Input: part model. Units: mm. Frame: model coordinates. Face numbers are marked on the shaded views. A direction names the side the tool comes from. Round coordinates to 2 decimals unless told otherwise and drop trailing zeros. Order: outer loops, then holes, each group sorted by start corner. A loop starts at its lowest first (then second) coordinate and runs counter-clockwise, first axis right, second up. Notation, with made-up numbers: (-22.5, -22) -> (-0.5, -22) arc R23 ccw to (-0.5, 13) -> close; hole circle Ø5 at (89.5, 81.5). An arc over 180 degrees is marked (long way). Use a Markdown table: item, result.
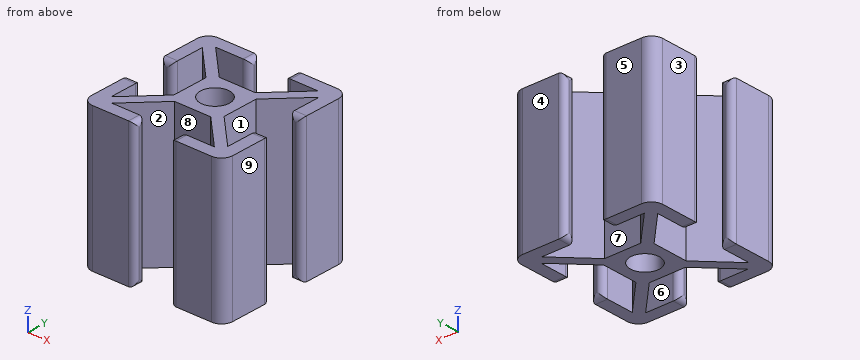
from build123d import *

# Parameters (mm, degrees)
SKETCH_W     = 25.4
SKETCH_H     = 25.4
SKETCH_R     = 2.6035
PAD_DEPTH    = 25.4
POCKET_DEPTH = 25.401
FILLET_R     = 1.0049
FILLET001_R  = 2


with BuildPart() as part:
    # Sketch → Pad (new body)
    with BuildSketch(Plane.XY):
        Rectangle(SKETCH_W, SKETCH_H)
        Circle(SKETCH_R, mode=Mode.SUBTRACT)
    extrude(amount=PAD_DEPTH)

    # Sketch001 (on Face7 of Pad) → Pocket (cut, through all)
    with BuildSketch(Plane.XY.offset(25.4)):
        Polygon((-3.2512, 12.7), (3.2512, 12.7), (3.2512, 10.4902), (9.2202, 10.4902), (3.2512, 4.5212), (-3.2512, 4.5212), (-9.2202, 10.4902), (-3.2512, 10.4902), align=None)
        Polygon((-4.5212, 3.2512), (-4.5212, -3.2512), (-10.4902, -9.2202), (-10.4902, -3.2512), (-12.7, -3.2512), (-12.7, 3.2512), (-10.4902, 3.2512), (-10.4902, 9.2202), align=None)
        Polygon((4.5212, 3.2512), (4.5212, -3.2512), (10.4902, -9.2202), (10.4902, -3.2512), (12.7, -3.2512), (12.7, 3.2512), (10.4902, 3.2512), (10.4902, 9.2202), align=None)
        Polygon((3.2512, -4.5212), (-3.2512, -4.5212), (-9.2202, -10.4902), (-3.2512, -10.4902), (-3.2512, -12.7), (3.2512, -12.7), (3.2512, -10.4902), (9.2202, -10.4902), align=None)
    extrude(amount=-POCKET_DEPTH, mode=Mode.SUBTRACT)

    # Fillet
    fillet_edges = [part.edges().sort_by_distance(p)[0] for p in [
        (-11.5951, 3.2512, 25.4),
        (-10.4902, 3.2512, 12.7),
        (-11.5951, 3.2512, 0),
        (-12.7, 3.2512, 12.7),
        (11.5951, 3.2512, 25.4),
        (10.4902, 3.2512, 12.7),
        (11.5951, 3.2512, 0),
        (12.7, 3.2512, 12.7),
        (11.5951, -3.2512, 25.4),
        (10.4902, -3.2512, 12.7),
        (11.5951, -3.2512, 0),
        (12.7, -3.2512, 12.7),
        (-11.5951, -3.2512, 25.4),
        (-10.4902, -3.2512, 12.7),
        (-11.5951, -3.2512, 0),
        (-12.7, -3.2512, 12.7),
        (-3.2512, 11.5951, 25.4),
        (-3.2512, 10.4902, 12.7),
        (-3.2512, 11.5951, 0),
        (-3.2512, 12.7, 12.7),
        (3.2512, 11.5951, 25.4),
        (3.2512, 10.4902, 12.7),
        (3.2512, 11.5951, 0),
        (3.2512, 12.7, 12.7),
        (-3.2512, -11.5951, 25.4),
        (-3.2512, -10.4902, 12.7),
        (-3.2512, -11.5951, 0),
        (-3.2512, -12.7, 12.7),
        (3.2512, -11.5951, 25.4),
        (3.2512, -10.4902, 12.7),
        (3.2512, -11.5951, 0),
        (3.2512, -12.7, 12.7),
    ]]
    fillet(fillet_edges, radius=FILLET_R)

    # Fillet001
    fillet001_edges = [part.edges().sort_by_distance(p)[0] for p in [
        (12.7, -12.7, 12.7),
        (12.7, 12.7, 12.7),
        (-12.7, -12.7, 12.7),
        (-12.7, 12.7, 12.7),
    ]]
    fillet(fillet001_edges, radius=FILLET001_R)


solid = part.part
1) Cut plane B-B on x = 0. Return loops of the section in (y, z), and give its area (3 significant figures).
Answer key:
| item | result |
|---|---|
| outline | (-4.52, 0) -> (-2.6, 0) -> (-2.6, 25.4) -> (-4.52, 25.4) -> close; (2.6, 0) -> (4.52, 0) -> (4.52, 25.4) -> (2.6, 25.4) -> close |
| area | 97.4 mm^2 |
2) Draft query along X for the marked faces 1, 2, 3 and 4. Return one class per face: released by +X, released by -X, zero draft, split by the parting line, or undercut.
Answer key:
| item | result |
|---|---|
| face 1 | released by +X |
| face 2 | undercut |
| face 3 | released by -X |
| face 4 | zero draft |
3) Cut plane A-A on y = 6. Return loops of the section in (x, z), and give its area (3 significant figures).
Answer key:
| item | result |
|---|---|
| outline | (-12.7, 0) -> (-10.49, 0) -> (-10.49, 25.4) -> (-12.7, 25.4) -> close; (-7.27, 0) -> (-4.73, 0) -> (-4.73, 25.4) -> (-7.27, 25.4) -> close; (4.73, 0) -> (7.27, 0) -> (7.27, 25.4) -> (4.73, 25.4) -> close; (10.49, 0) -> (12.7, 0) -> (12.7, 25.4) -> (10.49, 25.4) -> close |
| area | 241 mm^2 |
4) Ray query, probe 1 along Y at (x, z) = (0, 18); probe 2 along Y at (x, z) = (7, 22.5); probe 3 along Y at (x, z) = (6.75, 16.25). Return the intervals inside material, ascending.
Answer key:
| item | result |
|---|---|
| probe 1 | y = -4.52 to -2.6, 2.6 to 4.52 |
| probe 2 | y = -12.7 to -10.49, -8.27 to -5.73, 5.73 to 8.27, 10.49 to 12.7 |
| probe 3 | y = -12.7 to -10.49, -8.02 to -5.48, 5.48 to 8.02, 10.49 to 12.7 |
5) Set-up query: the marked faces 5, 6, 7, 8 and 9. Return all of +Z, -Z, +X, -X, +Y, -Y with unobstructed straight access to the full face (end or side cutting, diameter ignored); none if empty.
Answer key:
| item | result |
|---|---|
| face 5 | +Z, -Z, +X, -X, +Y |
| face 6 | +Z, -Z |
| face 7 | +Z, -Z, +Y |
| face 8 | +Z, -Z, -Y |
| face 9 | +Z, -Z, +X, +Y, -Y |
